from build123d import *

# Parameters (mm, degrees)
F0_W     = 95
F0_H     = 145
F1_DEPTH = 12
F2_W     = 26
F2_H     = 65
F3_DEPTH = 15
F4_W     = 26
F4_H     = 65
F5_DEPTH = 15


with BuildPart() as f1:
    # F0 (on Front) → F1 (new body)
    with BuildSketch(Plane.XZ):
        Rectangle(F0_W, F0_H)
    extrude(amount=-F1_DEPTH)

    # F2 (on face) → F3 (cut)
    with BuildSketch(Plane.XZ):
        with Locations((34.5, -40)):
            Rectangle(F2_W, F2_H)
    extrude(amount=-F3_DEPTH, mode=Mode.SUBTRACT)

    # F4 (on face) → F5 (cut)
    with BuildSketch(Plane.XZ):
        with Locations((-34.5, -40)):
            Rectangle(F4_W, F4_H)
    extrude(amount=-F5_DEPTH, mode=Mode.SUBTRACT)


solid = f1.part
Design review of the part built by this model. Coordinates are the model's own, in mm. A direction names the side the tool comes from. Round coordinates to 2 decimals unless told otherwise and drop trailing zeros. Order: outer loops, then holes, each group sorted by start corner. A loop starts at its lowest first (then second) coordinate and runs counter-clockwise, first axis right, second up.
1) Consider section A-A (y = 4.5). State the section outline as (x, z) points.
The answers:
outline: (-47.5, -7.5) - (-21.5, -7.5) - (-21.5, -72.5) - (21.5, -72.5) - (21.5, -7.5) - (47.5, -7.5) - (47.5, 72.5) - (-47.5, 72.5) - close
2) For L1, parallel to X at y = 3.5, z = -61.5; L2, parallel to Z at x = -42.5, y = 8, list the stretches that pass through material, from the lowest coordinate up.
The answers:
L1: x = -21.5 to 21.5
L2: z = -7.5 to 72.5
3) Consider section B-B (x = 40.5). State the section outline as (y, z) points, plus the area to 3 significant figures.
The answers:
outline: (0, -7.5) - (12, -7.5) - (12, 72.5) - (0, 72.5) - close
area: 960 mm2
4) Clearance check with flat-ended pins moving along their axes: pin 1 Ø3 at (x, y) = (-24, 4.5) entering from -Z; pin 2 Ø6 at (y, z) = (9.5, -49) entering from -X; pin 3 Ø3.5 at (y, z) = (4.5, -30.5) entering from +X. State where each tip first meets the part, or that it passes through.
The answers:
pin 1: stops at z = -7.5
pin 2: stops at x = -21.5
pin 3: stops at x = 21.5
5) Machinability: for faces 1 (the flat face through (-21.5, 6, -40)), 2 (the flat face through (21.5, 6, -40)), 3 (the flat face through (-47.5, 6, 32)), which of the approach directions +Z, -Z, +X, -X, +Y, -Y give a long, thin tool a straight path to every point of the face, cutting with its end or side? Answer none if there is none.
The answers:
face 1: -Z, -X, +Y, -Y
face 2: -Z, +X, +Y, -Y
face 3: +Z, -Z, -X, +Y, -Y
6) Consider section C-C (z = -24). State the section outline as (x, y) points, plus the area to 3 significant figures.
The answers:
outline: (-21.5, 0) - (21.5, 0) - (21.5, 12) - (-21.5, 12) - close
area: 516 mm2
